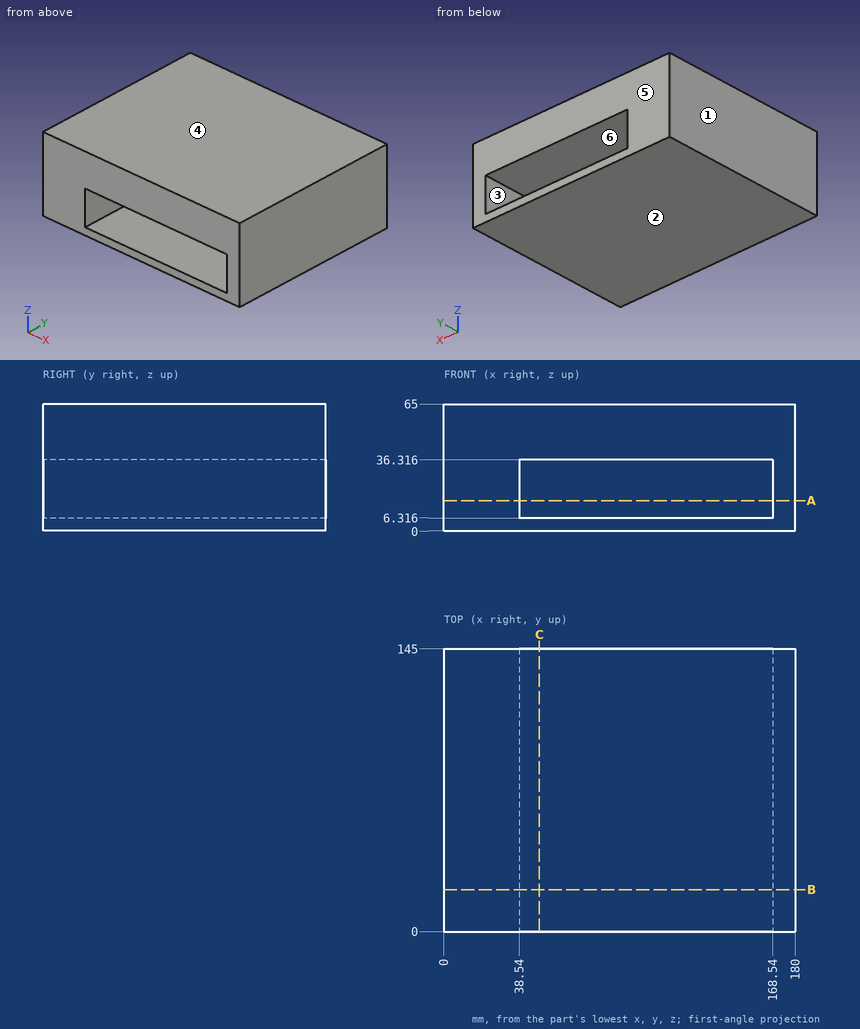
Geometry: see drawing. Coordinates: mm, zero at the bounding-box minimum. A direction names the side the tool comes from. Coordinates: 2 decimals unless noted, no trailing zeros. Write each loop counter-clockwise with the first axis right and the second up, starting at its lowest first coordinate (ties: lowest second). Pieces come first, ordered by that corner, then holes. Notation, with made-up numbers: M 25,54 L 76,54 A25 ccw 76,93 Z; hole C 85.25,35 d6. An arc over 180 degrees is marked long. Answer as a JSON object with one key per item and string values.
1. Cut plane C-C on x = 49. Output: boundary loops of the cut face in (y, z) (1 decimal).
Evaluation:
{"outline": "M 0,0 L 145,0 L 145,6.3 L 0,6.3 Z; M 0,36.3 L 145,36.3 L 145,65 L 0,65 Z"}
2. Access query for the marked faces 5 and 6. Directions: +Z, -Z, +X, -X, +Y, -Y. A direction counts if a zero-diameter tool reaches every point of the face in a straight line with its end or side. Return the directions, or none.
Evaluation:
{"face 5": "+Z, -Z, +X, -X, +Y", "face 6": "+Y, -Y"}
3. Cut plane B-B on y = 21.5. Output: boundary loops of the cut face in (x, z) (1 decimal).
Evaluation:
{"outline": "M 0,0 L 180,0 L 180,65 L 0,65 Z; hole M 38.5,6.3 L 168.5,6.3 L 168.5,36.3 L 38.5,36.3 Z"}
4. Draft query along Z for the marked faces 1, 2, 3 and 4. Return one class per face: released by +Z, released by -Z, zero draft, split by the parting line, or undercut.
Evaluation:
{"face 1": "zero draft", "face 2": "released by -Z", "face 3": "undercut", "face 4": "released by +Z"}
5. Cut plane A-A on z = 15.5. Output: boundary loops of the cut face in (x, y), plus the area to 3 significant figures.
Evaluation:
{"outline": "M 0,0 L 38.54,0 L 38.54,145 L 0,145 Z; M 168.54,0 L 180,0 L 180,145 L 168.54,145 Z", "area": "7,250 mm^2"}
6. Ray query, L1, parallel to X at y = 48.5, z = 11; L2, parallel to Z at x = 135.5, y = 97.5 (1 decimal). Return the intervals inside material, ascending.
Evaluation:
{"L1": "0 to 38.54, 168.54 to 180", "L2": "0 to 6.3, 36.3 to 65"}
